Read the model definition and answer for the solid it produces. Units are mm, in the model's axes. Give positions to 0.01 mm unless a question says otherwise; leave off trailing zeros. Write each loop counter-clockwise with the first axis right and the second up, starting at its lowest first coordinate (ties: lowest second). Pieces come first, ordered by that corner, then holes. Notation, with made-up numbers: (-32, 22) - (16, 22) arc R20 ccw to (16, 58) - close; hole circle Ø8 at (-8, 43.5). An arc over 180 degrees is marked (long way). Answer as a JSON object with one key per item and string values. Group by question number.
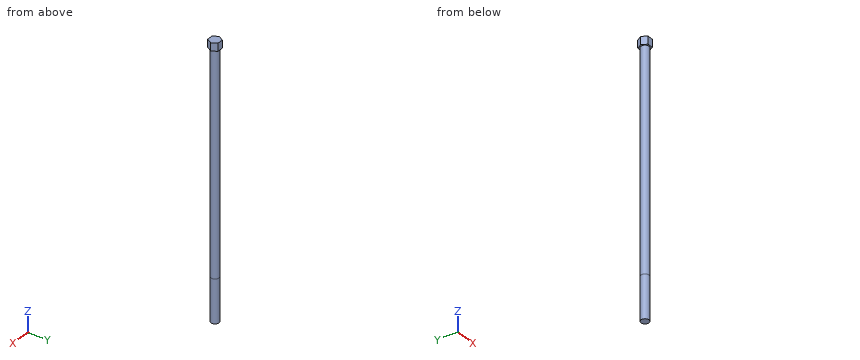
```python
from build123d import *

# Parameters (mm, degrees)
SKETCH_1_R      = 5
EXTRUDE_1_DEPTH = 280
EXTRUDE_2_DEPTH = 10
EXTRUDE_START   = 55
SKETCH_3_R      = 5
EXTRUDE_3_DEPTH = 55


with BuildPart() as part:
    # 草图1 → 凸台-拉伸1 (new body)
    with BuildSketch(Plane.XY):
        Circle(SKETCH_1_R)
    extrude(amount=EXTRUDE_1_DEPTH)

    # 草图2 → 凸台-拉伸2 (add)
    with BuildSketch(Plane.XY.offset(280)):
        Polygon((3.75, -6.495190528), (7.5, 0), (3.75, 6.495190528), (-3.75, 6.495190528), (-7.5, 0), (-3.75, -6.495190528), align=None)
    extrude(amount=EXTRUDE_2_DEPTH)

    # 草图3 → 凸台-拉伸3 (add)
    with BuildSketch(Plane(origin=(0, 0, 0), x_dir=(-1, 0, 0), z_dir=(0, 0, -1)).offset(EXTRUDE_START)):
        Circle(SKETCH_3_R)
    extrude(amount=-EXTRUDE_3_DEPTH)


solid = part.part
```
1) Flat-ended cylindrical pins translate along their axes: pin 1 Ø8 at (x, z) = (-5.5, 50.5) entering from +Y; pin 2 Ø2 at (x, z) = (3.5, 103) entering from +Y; pin 3 Ø3 at (x, z) = (-1, 184.5) entering from -Y. Find the tip coordinate at first contact, or state that the pin passes through.
2) Find the intervals of material crossed by line 1 (Z direction, x = -2.75, y = -5); line 2 (X direction, y = -0.25, z = 103), in increasing order. Write a range as [from, to].
3) Find section B-B, the plane z = 15.5. Write down the section's boundary in (x, y).
4) Find section A-A, the plane x = 0. Write down the section's boundary in (y, z), and give its area (3 significant figures).
Values follow:
{
 "1": {"pin 1": "stops at y = 4.77", "pin 2": "stops at y = 4.33", "pin 3": "stops at y = -5"},
 "2": {"line 1": "z = [280, 290]", "line 2": "x = [-4.99, 4.99]"},
 "3": {"outline": "circle Ø10 at (0, 0)"},
 "4": {"outline": "(-6.5, 280) - (-5, 280) - (-5, -55) - (5, -55) - (5, 280) - (6.5, 280) - (6.5, 290) - (-6.5, 290) - close", "area": "3,480 mm2"}
}
